Could you check a few things on this model? Use its own coordinates, in mm. A direction names the side the tool comes from. Round coordinates to 2 decimals unless told otherwise and drop trailing zeros. Write each loop counter-clockwise with the first axis right and the second up, starting at its lowest first coordinate (ties: lowest second). Pieces come first, ordered by that corner, then holes. Notation, with made-up numbers: (-3.75, 40.25) -> (42.25, 40.25) arc R17 ccw to (42.25, 73.25) -> close; hole circle Ø1 at (-23.5, 44). An arc over 180 degrees is marked (long way). One line per question, with ' | ' between items. Start each with the question number.
1. For pin 1 Ø3 at (y, z) = (86.5, 0.5) entering from +X; pin 2 Ø6.5 at (x, y) = (2.5, 62.5) entering from -Z; pin 3 Ø7.5 at (y, z) = (63, 6) entering from -X, each with a flat end and sliding along its axis, tell me the tip position at first contact or that it passes through.
2. Imagine slicing it at C-C, the plane z = -7. List the corners of the cut face in (x, y) for me (3 decimals), and give its area (3 significant figures).
3. If I drill on line 1 along Z through (x, y) = (1, 148) (3 decimals); line 2 along Z through (x, y) = (5, 59.5) (3 decimals), over which ranges is the centre line in solid material (lowest first)? Write a range as [from, to].
4. For faces 4 (the flat face through (0, 95, 10.795)), 5 (the flat face through (0, 119, -12.7)), 6 (the flat face through (21, 161, 12.7)), 7 (the flat face through (13.1, 217.24, -6.21)), 8 (the flat face through (-12.7, 113, 0)), which set-ups out of +Z, -Z, +X, -X, +Y, -Y let a thin tool reach every point of the face, with its end or its side?
5. Imagine slicing it at B-B, the plane y = 213.5. List the corners of the cut face in (x, z) for me (3 decimals), and give its area (3 significant figures).
6. Imagine slicing it at D-D, the plane x = 4.5. List the corners of the cut face in (y, z) for me (3 decimals), and give its area (3 significant figures).
7. Thinking about a two-plate mould opening in Z: for faces 1 (the cylindrical face through (-11.76, 5.41, 0.69)), 2 (the flat face through (0, 75, 12.7)), 3 (the flat face through (-28.575, 196.4, 6.2)), which applies, released by +Z, released by -Z, zero draft, split by the parting line, or undercut?
8. Imagine slicing it at A-A, the plane x = 18. List the corners of the cut face in (y, z) for me, and give its area (3 significant figures).
from build123d import *

# Parameters (mm, degrees)
SKETCH1_W               = 25.4
SKETCH1_H               = 25.4
SKETCH1_W_2             = 21.59
SKETCH1_H_2             = 21.59
BOSS_EXTRUDE1_DEPTH     = 228.6
CUT_EXTRUDE1_DEPTH      = 230.304470083
CUT_EXTRUDE1_DEPTH_BACK = 230.304470083
SKETCH2_R               = 3.175
BOSS_EXTRUDE2_DEPTH     = 28.575
FILLET1_R               = 7.62


with BuildPart() as part:
    # Sketch1 → Boss-Extrude1 (new body)
    with BuildSketch(Plane(origin=(0, 0, 0), x_dir=(1, 0, 0), z_dir=(0, 1, 0))):
        Rectangle(SKETCH1_W, SKETCH1_H)
        Rectangle(SKETCH1_W_2, SKETCH1_H_2, mode=Mode.SUBTRACT)
    extrude(amount=BOSS_EXTRUDE1_DEPTH)

    # Sketch2 → Cut-Extrude1 (cut, two sides: drawn at the far end of the back side and taken through both)
    with BuildSketch(Plane(origin=(0, 0, 0), x_dir=(0, 0, -1), z_dir=(1, 0, 0)).offset(-CUT_EXTRUDE1_DEPTH_BACK)):
        Polygon((-12.7, 228.6), (-12.7, 184.15), (12.7, 228.6), align=None)
        with BuildLine():
            Line((-12.7, 0), (0, 0))
            ThreePointArc((0, 0), (-8.980256121, 3.719743879), (-12.7, 12.7))
            Line((-12.7, 12.7), (-12.7, 0))
        make_face()
        with BuildLine():
            ThreePointArc((12.7, 12.7), (8.980256121, 3.719743879), (0, 0))
            Line((0, 0), (12.7, 0))
            Line((12.7, 0), (12.7, 12.7))
        make_face()
        with Locations((0, 8.509)):
            Circle(SKETCH2_R)
    extrude(amount=CUT_EXTRUDE1_DEPTH + CUT_EXTRUDE1_DEPTH_BACK, mode=Mode.SUBTRACT)

    # Sketch3 → Boss-Extrude2 (add, symmetric)
    with BuildSketch(Plane(origin=(0, 0, 0), x_dir=(0, 0, -1), z_dir=(1, 0, 0))):
        Polygon((-12.7, 184.15), (18.604025134, 238.932043985), (17.280822586, 239.688159727), (-14.224, 184.554720202), (-14.224, 138.834720202), (-12.7, 138.834720202), align=None)
    extrude(amount=BOSS_EXTRUDE2_DEPTH, both=True)

    # Fillet1
    fillet1_edges = [part.edges().sort_by_distance(p)[0] for p in [
        (-28.575, 239.310101856, -17.94242386),
        (-28.575, 138.834720202, 13.462),
        (28.575, 239.310101856, -17.94242386),
        (28.575, 138.834720202, 13.462),
    ]]
    fillet(fillet1_edges, radius=FILLET1_R)


solid = part.part
Geometry results:
1) pin 1: stops at x = 12.7 | pin 2: stops at z = -12.7 | pin 3: stops at x = -12.7
2) outline: (-28.575, 218.625) -> (-12.7, 218.625) -> (-12.7, 2.103) -> (-10.795, 2.103) -> (-10.795, 218.625) -> (10.795, 218.625) -> (10.795, 2.103) -> (12.7, 2.103) -> (12.7, 218.625) -> (28.575, 218.625) -> (28.575, 221.697) -> (-28.575, 221.697) -> close | area: 1,000 mm2
3) line 1: z = [-12.7, -10.795], [10.795, 14.224] | line 2: z = [-12.7, -10.795], [10.795, 12.7]
4) face 4: -Y | face 5: -Z, +X, -X, -Y | face 6: -Z, +X, -Y | face 7: -Z, -Y | face 8: -Z, -X, -Y
5) outline: (-28.575, -4.071) -> (-12.7, -4.071) -> (-12.7, -12.7) -> (12.7, -12.7) -> (12.7, -4.071) -> (28.575, -4.071) -> (28.575, -2.316) -> (-28.575, -2.316) -> close; hole (-10.795, -10.795) -> (10.795, -10.795) -> (10.795, -4.071) -> (-10.795, -4.071) -> close | area: 174 mm2
6) outline: (6.01, -10.795) arc R12.7 ccw to (12.7, -12.7) -> (228.6, -12.7) -> (238.932, -18.604) -> (239.688, -17.281) -> (184.555, 14.224) -> (138.835, 14.224) -> (138.835, 12.7) -> (12.7, 12.7) arc R12.7 ccw to (6.01, 10.795) -> (187.484, 10.795) -> (225.266, -10.795) -> close | area: 921 mm2
7) face 1: undercut | face 2: released by +Z | face 3: zero draft
8) outline: (138.83, 12.7) -> (184.15, 12.7) -> (238.93, -18.6) -> (239.69, -17.28) -> (184.55, 14.22) -> (138.83, 14.22) -> close | area: 166 mm2
